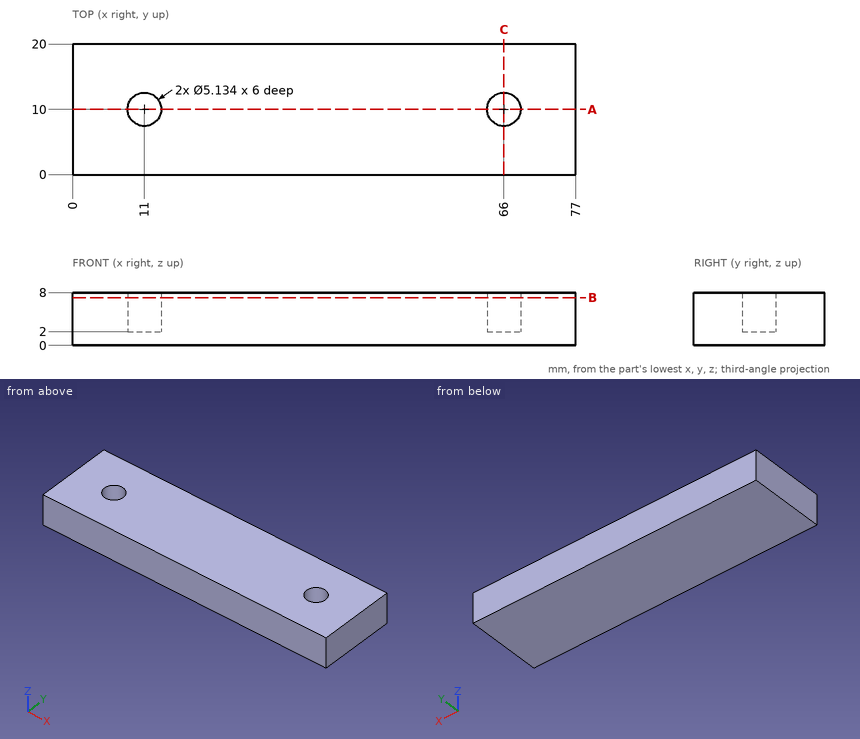
Geometry: see drawing. Coordinates: mm, zero at the bounding-box minimum. Round coordinates to 2 decimals unless told otherwise and drop trailing zeros. Loops run counter-clockwise (first coordinate to the right, second up) from the corner with the lowest first, then second, coordinate; pieces in that order, holes last. Notation, with made-up numbers: M -35,-10 L 19,-10 A31 cw 19,29 Z; hole C 60.5,87 d2. An arc over 180 degrees is marked long. Use a Markdown table: item, result. Add a question column.
1. Section query B-B on z = 7.25. Return the cut outline in (x, y).
2. Line query: line 1 (X direction, y = 10, z = 4.5); line 2 (Y direction, x = 11, z = 4.75); line 3 (X direction, y = 12, z = 6.5). Output: solid intervals per line, ascending.
3. Section query C-C on x = 66. Return the cut outline in (y, z).
4. Section query A-A on y = 10. Return the cut outline in (x, z), then the cut area to 3 significant figures.
5. Contact query for flat-ended pins moving along their axis: P1, Ø4, axis at x = 11, y = 10, coming from the -Z side; P2, Ø3, axis at x = 66, y = 10, coming from the +Z side. Output: stop coordinate, or through.
Reported:
| question | item | result |
|---|---|---|
| 1 | outline | M 0,0 L 77,0 L 77,20 L 0,20 Z; hole C 11,10 d5.13; hole C 66,10 d5.13 |
| 2 | line 1 | x = 0 to 8.43, 13.57 to 63.43, 68.57 to 77 |
| 2 | line 2 | y = 0 to 7.43, 12.57 to 20 |
| 2 | line 3 | x = 0 to 9.39, 12.61 to 64.39, 67.61 to 77 |
| 3 | outline | M 0,0 L 20,0 L 20,8 L 12.57,8 L 12.57,2 L 7.43,2 L 7.43,8 L 0,8 Z |
| 4 | outline | M 0,0 L 77,0 L 77,8 L 68.57,8 L 68.57,2 L 63.43,2 L 63.43,8 L 13.57,8 L 13.57,2 L 8.43,2 L 8.43,8 L 0,8 Z |
| 4 | area | 554 mm² |
| 5 | P1 | stops at z = 0 |
| 5 | P2 | stops at z = 2 |
